Check sheet for the drawn part. Datum: minimum x, y, z corner. Units: mm. A direction names the side the tool comes from. Give positions to 0.01 mm unless a question says otherwise; leave off trailing zeros. Write each loop counter-clockwise with the first axis right and the second up, starting at its lowest first coordinate (ties: lowest second). Pieces come first, ordered by that corner, then holes. Notation, with made-up numbers: (-33, -17.5) - (-19, -17.5) arc R27 ccw to (-19, 20.5) - close; hole circle Ø4 at (88.5, -35). An arc over 180 degrees is marked (long way). Use a Markdown table: item, result.
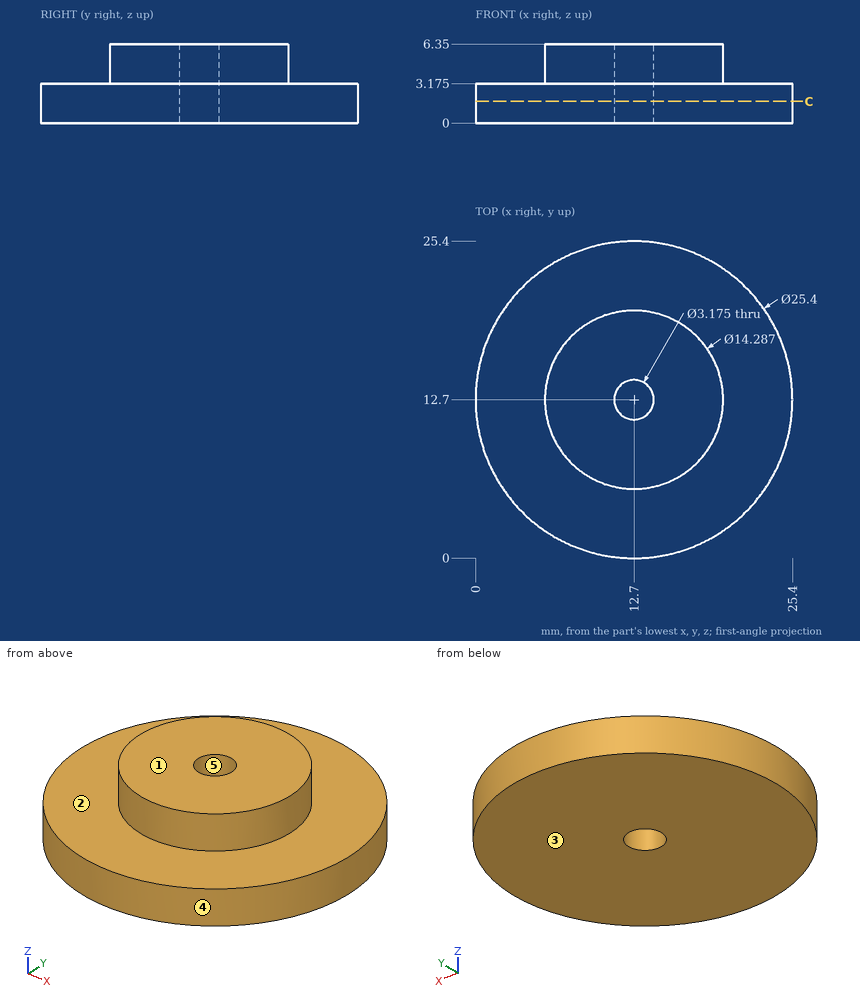
1) Depth check by flat-ended pin: P1, Ø2, axis at y = 14, z = 1.5, coming from the -X side; P2, Ø1.5, axis at x = 5.5, z = 1, coming from the +Y side; P3, Ø1, axis at x = 6.5, z = 4.5, coming from the +Y side (1 decimal). Enter the tip coordinate at first touch or a pass-through.
Working result:
| item | result |
|---|---|
| P1 | stops at x = 0 |
| P2 | stops at y = 23.64 |
| P3 | stops at y = 17 |
2) Material ranges on L1, parallel to Y at x = 12.7, z = 3.5; L2, parallel to Y at x = 12.7, z = 1.5; L3, parallel to Z at x = 23.25, y = 12 (1 decimal), recorded low to high. Write a range as from..to.
Working result:
| item | result |
|---|---|
| L1 | y = 5.56..11.11, 14.29..19.84 |
| L2 | y = 0..11.11, 14.29..25.4 |
| L3 | z = 0..3.2 |
3) Mould release check, pull along X, two halves, no side actions. Record for the marked faces 3, 4 and 5: pulls with the +X half, pulls with the -X half, needs draft (parallel to the pull), parting line crosses it, or undercut.
Working result:
| item | result |
|---|---|
| face 3 | needs draft |
| face 4 | parting line crosses it |
| face 5 | undercut |
4) Set-up check for the marked faces 1 and 2: record each of +Z, -Z, +X, -X, +Y, -Y from which the full face is reachable in a straight line by a thin tool's end or side.
Working result:
| item | result |
|---|---|
| face 1 | +Z, +X, -X, +Y, -Y |
| face 2 | +Z |
5) Section check C-C on z = 1.75. Record the boundary of the cut face in (x, y) (1 decimal), then the cut area to 3 significant figures.
Working result:
| item | result |
|---|---|
| outline | circle Ø25.4 at (12.7, 12.7); hole circle Ø3.2 at (12.7, 12.7) |
| area | 499 mm² |
